For this review, use the dimensioned drawing (mm, ordinates from the lowest corner) and the shaded views. A direction names the side the tool comes from. Give positions to 0.01 mm unless a question says otherwise; leave off trailing zeros. Loops run counter-clockwise (first coordinate to the right, second up) from the corner with the lowest first, then second, coordinate; pieces in that order, holes last. Notation, with made-up numbers: (-1, 11) -> (33, 11) arc R25 ccw to (33, 46) -> close; hole circle Ø11 at (-10, -4.75). An arc over 180 degrees is marked (long way). Write each question's results on one line, items separated by ' | '. Start each with the question number.
Q1. We need section B-B (y = 35). Write out the cut boundary in (x, z), plus the area to 3 significant figures.
Q2. Wall thickness on L1, parallel to X at y = 11.5, z = 2.5; L2, parallel to Z at x = 193, y = 35; L3, parallel to Y at x = 256, z = 15.5: over which ranges is each line inside the solid? List them lowest first. Write a range as [from, to].
Q3. Insertion check: pin 1 Ø4 at (x, z) = (191.5, 20) entering from -Y; pin 2 Ø10 at (x, y) = (240, 44) entering from -Z; pin 3 Ø6 at (y, z) = (11, 19) entering from -X. Each pin has a flat end and moves straight along its axis. Give the tip position at first contact, or say it passes through.
Q4. Machinability: for the marked faces 1, 2 and 3, which of the approach directions +Z, -Z, +X, -X, +Y, -Y give a long, thin tool a straight path to every point of the face, cutting with its end or side? Answer none if there is none.
Q5. We need section C-C (y = 11.5). Write out the cut boundary in (x, z).
Q6. We need section A-A (z = 20). Write out the cut boundary in (x, y), plus the area to 3 significant figures.
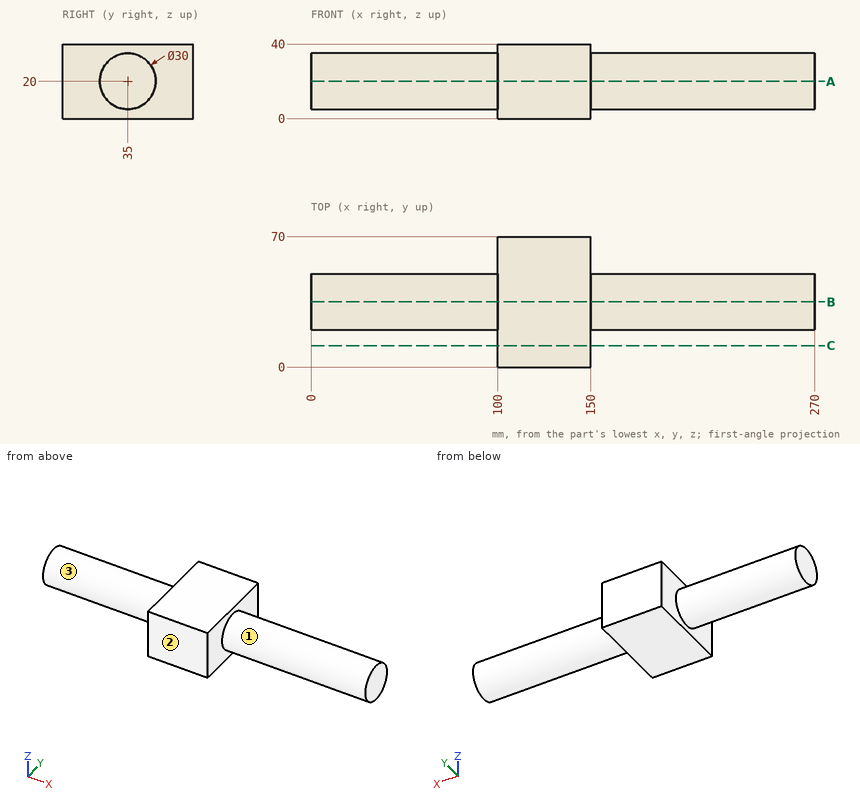
Output:
1) outline: (0, 5) -> (100, 5) -> (100, 0) -> (150, 0) -> (150, 5) -> (270, 5) -> (270, 35) -> (150, 35) -> (150, 40) -> (100, 40) -> (100, 35) -> (0, 35) -> close | area: 8,600 mm2
2) L1: [100, 150] | L2: [5, 35] | L3: [20.69, 49.31]
3) pin 1: y = 20 | pin 2: z = 5.54 | pin 3: x = 100
4) face 1: +X | face 2: +Z, -Z, +X, -X, -Y | face 3: -X
5) outline: (100, 0) -> (150, 0) -> (150, 40) -> (100, 40) -> close
6) outline: (0, 20) -> (100, 20) -> (100, 0) -> (150, 0) -> (150, 20) -> (270, 20) -> (270, 50) -> (150, 50) -> (150, 70) -> (100, 70) -> (100, 50) -> (0, 50) -> close | area: 10,100 mm2
